For this review, take the finished solid that the model builds, in its own axes (mm). Round coordinates to 2 decimals unless told otherwise and drop trailing zeros. Write each loop counter-clockwise with the first axis right and the second up, starting at its lowest first coordinate (ties: lowest second). Pieces come first, ordered by that corner, then holes.
from build123d import *

# Parameters (mm, degrees)
SKETCH021_W     = 116.5
SKETCH021_H     = 84
PAD008_DEPTH    = 2
SKETCH022_W     = 112.5
SKETCH022_H     = 80
PAD009_DEPTH    = 2
SKETCH023_W     = 108.5
SKETCH023_H     = 76
POCKET013_DEPTH = 2
FILLET014_R     = 1
FILLET015_R     = 1
FILLET016_R     = 1
FILLET017_R     = 1
FILLET018_R     = 1
FILLET019_R     = 1
FILLET020_R     = 1
FILLET021_R     = 0.5
FILLET022_R     = 1
FILLET023_R     = 1


with BuildPart() as part:
    # Sketch021 → Pad008 (new body)
    with BuildSketch(Plane(origin=(0, 0, 0), x_dir=(1, 0, 0), z_dir=(0, 0, -1))):
        with Locations((58.25, 42)):
            Rectangle(SKETCH021_W, SKETCH021_H)
    extrude(amount=PAD008_DEPTH)

    # Sketch022 (on Face5 of Pad008) → Pad009 (new body)
    with BuildSketch(Plane.XY):
        with Locations((58.25, -42)):
            Rectangle(SKETCH022_W, SKETCH022_H)
    extrude(amount=PAD009_DEPTH)

    # Sketch023 (on Face11 of Pad009) → Pocket013 (cut)
    with BuildSketch(Plane.XY.offset(2)):
        with Locations((58.25, -42)):
            Rectangle(SKETCH023_W, SKETCH023_H)
    extrude(amount=-POCKET013_DEPTH, mode=Mode.SUBTRACT)

    # Fillet014
    fillet014_edges = [part.edges().sort_by_distance(p)[0] for p in [
        (114.5, -82, 1),
    ]]
    fillet(fillet014_edges, radius=FILLET014_R)

    # Fillet015
    fillet015_edges = [part.edges().sort_by_distance(p)[0] for p in [
        (114.5, -2, 1),
        (116.5, 0, -1),
    ]]
    fillet(fillet015_edges, radius=FILLET015_R)

    # Fillet016
    fillet016_edges = [part.edges().sort_by_distance(p)[0] for p in [
        (116.5, -84, -1),
    ]]
    fillet(fillet016_edges, radius=FILLET016_R)

    # Fillet017
    fillet017_edges = [part.edges().sort_by_distance(p)[0] for p in [
        (0, -84, -1),
        (2, -82, 1),
    ]]
    fillet(fillet017_edges, radius=FILLET017_R)

    # Fillet018
    fillet018_edges = [part.edges().sort_by_distance(p)[0] for p in [
        (0, 0, -1),
        (2, -2, 1),
    ]]
    fillet(fillet018_edges, radius=FILLET018_R)

    # Fillet019
    fillet019_edges = [part.edges().sort_by_distance(p)[0] for p in [
        (58.25, -4, 2),
    ]]
    fillet(fillet019_edges, radius=FILLET019_R)

    # Fillet020
    fillet020_edges = [part.edges().sort_by_distance(p)[0] for p in [
        (4, -42, 2),
    ]]
    fillet(fillet020_edges, radius=FILLET020_R)

    # Fillet021
    fillet021_edges = [part.edges().sort_by_distance(p)[0] for p in [
        (58.25, -2, 2),
    ]]
    fillet(fillet021_edges, radius=FILLET021_R)

    # Fillet022
    fillet022_edges = [part.edges().sort_by_distance(p)[0] for p in [
        (58.25, -80, 2),
    ]]
    fillet(fillet022_edges, radius=FILLET022_R)

    # Fillet023
    fillet023_edges = [part.edges().sort_by_distance(p)[0] for p in [
        (112.5, -42, 2),
    ]]
    fillet(fillet023_edges, radius=FILLET023_R)


solid = part.part
(1) For pin 1 Ø1.2 at (x, z) = (82.5, 1) entering from -Y; pin 2 Ø1.6 at (x, z) = (68, 0.5) entering from +Y; pin 3 Ø1 at (y, z) = (-22.5, 1) entering from +X; pin 4 Ø0.8 at (y, z) = (-36, 1) entering from -X, all flat-tipped, find the tip position at first contact; note any pin that passes through.
Geometry check:
pin 1: stops at y = -82
pin 2: stops at y = 0
pin 3: stops at x = 114.5
pin 4: stops at x = 2
(2) We need section A-A, the plane x = 62. Give the boundary of the cut face in (y, z), and give its area (3 significant figures).
Geometry check:
outline: (-84, -2) - (0, -2) - (0, 0) - (-2, 0) - (-2, 1.5) arc R0.5 ccw to (-2.5, 2) - (-3, 2) arc R1 ccw to (-4, 1) - (-4, 0) - (-80, 0) - (-80, 1) arc R1 ccw to (-81, 2) - (-81.5, 2) arc R0.5 ccw to (-82, 1.5) - (-82, 0) - (-84, 0) - close
area: 175 mm2
(3) Mouldability with a two-part tool opening along Y and no side actions: class faces 1 (the face through (57, -43, -2)), 2 (the face through (57, -41, 0)) as pulls with the +Y half, pulls with the -Y half, needs draft (parallel to the pull), parting line crosses it, or undercut.
Geometry check:
face 1: needs draft
face 2: undercut
(4) We need section B-B, the plane y = -9. Give the boundary of the cut face in (x, z).
Geometry check:
outline: (0, -2) - (116.5, -2) - (116.5, 0) - (114.5, 0) - (114.5, 1.5) arc R0.5 ccw to (114, 2) - (113.5, 2) arc R1 ccw to (112.5, 1) - (112.5, 0) - (4, 0) - (4, 1) arc R1 ccw to (3, 2) - (2.5, 2) arc R0.5 ccw to (2, 1.5) - (2, 0) - (0, 0) - close
(5) For line 1 along X through (y, z) = (-49.5, 0.85); line 2 along Z through (x, y) = (70, -50); line 3 along Y through (x, z) = (47, 1.4), list the stretches that pass through material, from the lowest coordinate up.
Geometry check:
line 1: x = 2 to 4, 112.5 to 114.5
line 2: z = -2 to 0
line 3: y = -82 to -80.08, -3.92 to -2
